```python
from build123d import *

# Parameters (mm, degrees)
CROQUIS1_W                   = 22
CROQUIS1_H                   = 6.35
SALIENTE_EXTRUIR1_DEPTH      = 2.8067
SALIENTE_EXTRUIR2_REACH      = 24.404
SALIENTE_EXTRUIR2_END_RADIUS = 3.9624
CORTAR_EXTRUIR1_DEPTH        = 23.404423445


with BuildPart() as part:
    # Croquis1 → Saliente-Extruir1 (new body)
    with BuildSketch(Plane(origin=(0, 0, 0), x_dir=(1, 0, 0), z_dir=(0, 1, 0))):
        Rectangle(CROQUIS1_W, CROQUIS1_H)
    extrude(amount=SALIENTE_EXTRUIR1_DEPTH)

    # Saliente-Extruir2: up to this cylinder (the profile starts outside it)
    saliente_extruir2_end = Plane(origin=(-15.73075, 1.120248, 0), z_dir=(0, -1, 0)) * Cylinder(SALIENTE_EXTRUIR2_END_RADIUS, 57.7328, mode=Mode.PRIVATE)
    # Croquis2 → Saliente-Extruir2 (add, up to the surface)
    with BuildSketch(Plane.ZY.offset(11), mode=Mode.PRIVATE) as saliente_extruir2_sk1:
        Polygon((1.35, 1.152803077), (0.692307692, 1.152803077), (0.692307692, 2.329726154), (0.346153846, 2.329726154), (-1.315384615, 1.048956923), (-1.315384615, 0.806649231), (0.346153846, 0.806649231), (0.346153846, 0.460495385), (0.692307692, 0.460495385), (0.692307692, 0.806649231), (1.35, 0.806649231), align=None)
        Polygon((0.346153846, 1.152803077), (-0.626322115, 1.152803077), (0.346153846, 1.9024425), align=None, mode=Mode.SUBTRACT)
    saliente_extruir2_tool1 = extrude(saliente_extruir2_sk1.sketch, amount=SALIENTE_EXTRUIR2_REACH, mode=Mode.PRIVATE) - saliente_extruir2_end
    add(saliente_extruir2_tool1.solids().sort_by_distance((-11, 1.120248, 1.021154))[0])

    # Croquis5 → Cortar-Extruir1 (cut, through all)
    # profile 1 of 2: a face of its own
    with BuildSketch(Plane.ZY.offset(11)):
        Polygon((1.35, 1.152803077), (1.35, 0.806649231), (0.692307692, 0.806649231), (0.692307692, 0.460495385), (0.346153846, 0.460495385), (0.346153846, 0.806649231), (-1.315384615, 0.806649231), (-1.315384615, 1.048956923), (0.346153846, 2.329726154), (0.692307692, 2.329726154), (0.692307692, 1.152803077), align=None)
        Polygon((0.578007692, 0.920949231), (1.2357, 0.920949231), (1.2357, 1.038503077), (0.578007692, 1.038503077), (0.578007692, 2.215426154), (0.385093942, 2.215426154), (-1.201084615, 0.992746849), (-1.201084615, 0.920949231), (0.460453846, 0.920949231), (0.460453846, 0.574795385), (0.578007692, 0.574795385), align=None, mode=Mode.SUBTRACT)
    # profile 2 of 2: a face of its own
    with BuildSketch(Plane.ZY.offset(11)):
        Polygon((0.460453846, 2.13486934), (-0.961816385, 1.038503077), (0.460453846, 1.038503077), align=None)
        Polygon((0.346153846, 1.9024425), (-0.626322115, 1.152803077), (0.346153846, 1.152803077), align=None, mode=Mode.SUBTRACT)
    extrude(amount=CORTAR_EXTRUIR1_DEPTH, mode=Mode.SUBTRACT)


solid = part.part
```
Source: CAD feature listing. Evaluate the final solid. Frame: model axes, mm. Give positions to 0.01 mm unless a question says otherwise; leave off trailing zeros. Order: outer loops, then holes, each group sorted by start corner. A loop starts at its lowest first (then second) coordinate and runs counter-clockwise, first axis right, second up.
(1) Pull-direction query (Z, two-part tool) for faces 1 (the face through (0, 1, -3.175)), 2 (the face through (11, 1, 0)), 3 (the face through (-11, 1.4, 0.1)); classes: +Z half, -Z half, draft (parallel to the pull), parting line (faces both ways), or undercut.
(2) Contact query for flat-ended pins moving along their axis: P1, Ø0.5, axis at x = -11.5, z = -0.5, coming from the -Y side; P2, Ø0.7, axis at x = -11.5, z = 0, coming from the +Y side; P3, Ø1.5, axis at y = 2, z = 0.5, coming from the -X side. Output: stop coordinate, or through.
(3) Material intervals for line 1 along X through (y, z) = (2.5, 2.25); line 2 along X through (y, z) = (1.95, 0.5), sorted ascending.
(4) Section query C-C (y = 2.6). Return the cut outline in (x, z) (3 decimals), plus the area to 3 significant figures.
(5) Section query D-D (z = -0.25). Return the cut outline in (x, y).
(6) Section query A-A (y = 1.55). Return the cut outline in (x, z) (3 decimals), plus the area to 3 significant figures.
(7) Section query B-B (z = 2.75). Return the cut outline in (x, y), plus the area to 3 significant figures.
Outcome:
1. face 1: -Z half
1. face 2: draft
1. face 3: undercut
2. P1: stops at y = 0.92
2. P2: stops at y = 2.19
2. P3: stops at x = -11.81
3. line 1: x = -11 to 11
3. line 2: x = -11.8 to 11
4. outline: (-11, -3.175) - (11, -3.175) - (11, 3.175) - (-11, 3.175) - close
4. area: 140 mm2
5. outline: (-11.78, 0.92) - (-11, 0.92) - (-11, 0) - (11, 0) - (11, 2.81) - (-11, 2.81) - (-11, 1.73) - (-11.78, 1.73) - (-11.78, 1.59) - (-11, 1.59) - (-11, 1.04) - (-11.78, 1.04) - close
6. outline: (-11.811, 0.578) arc R3.962 cw to (-11.795, 0.46) - (-11, 0.46) - (-11, -0.298) - (-11.78, -0.298) arc R3.962 cw to (-11.797, -0.478) - (-11, -0.478) - (-11, -3.175) - (11, -3.175) - (11, 3.175) - (-11, 3.175) - (-11, 0.578) - close
6. area: 140 mm2
7. outline: (-11, 0) - (11, 0) - (11, 2.81) - (-11, 2.81) - close
7. area: 61.7 mm2
